Input: part model. Units: mm. Frame: model coordinates. Face numbers are marked on the shaded views. A direction names the side the tool comes from. Give positions to 0.01 mm unless a question says otherwise; leave off trailing zeros. Loops run counter-clockwise (first coordinate to the right, second up) from the corner with the lowest first, then second, coordinate; pieces in that order, holes last. Notation, with made-up numbers: (69.5, -36) -> (94.5, -36) arc R8 cw to (94.5, -26) -> close; hole circle Ø11 at (38.5, 25). An arc over 180 degrees is marked (long way). One line per question, with ' | ' between items.
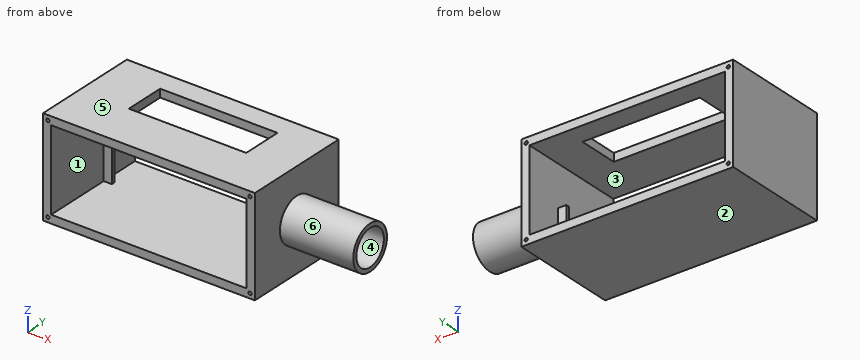
from build123d import *

# Parameters (mm, degrees)
SKETCH1_W           = 130
SKETCH1_H           = 60
BOSS_EXTRUDE1_DEPTH = 67
CUT_EXTRUDE1_REACH  = 69
SKETCH2_W           = 120
SKETCH2_H           = 50
SKETCH4_W           = 27.738428507
SKETCH4_H           = 2
BOSS_EXTRUDE2_DEPTH = 5
SKETCH5_W           = 27.5
SKETCH5_H           = 2
BOSS_EXTRUDE3_DEPTH = 5
CUT_EXTRUDE2_REACH  = 62
SKETCH6_W           = 72
SKETCH6_H           = 25
CUT_EXTRUDE3_REACH  = 69
SKETCH8_R           = 1
SKETCH9_R           = 13.5
BOSS_EXTRUDE4_DEPTH = 45
SKETCH10_R          = 11
CUT_EXTRUDE4_DEPTH  = 45


with BuildPart() as part:
    # Sketch1 → Boss-Extrude1 (new body)
    with BuildSketch(Plane(origin=(0, 0, 0), x_dir=(1, 0, 0), z_dir=(0, 1, 0))):
        Rectangle(SKETCH1_W, SKETCH1_H)
    extrude(amount=BOSS_EXTRUDE1_DEPTH)

    # Sketch2 → Cut-Extrude1 (cut, up to next)
    with BuildSketch(Plane(origin=(0, 67, 0), x_dir=(1, 0, 0), z_dir=(0, 1, 0)), mode=Mode.PRIVATE) as cut_extrude1_sk1:
        Rectangle(SKETCH2_W, SKETCH2_H)
    cut_extrude1_tool1 = extrude(cut_extrude1_sk1.sketch, amount=-CUT_EXTRUDE1_REACH, mode=Mode.PRIVATE) & part.part
    add(cut_extrude1_tool1.solids().sort_by_distance((0, 67, 0))[0], mode=Mode.SUBTRACT)

    # Sketch4 → Boss-Extrude2 (add)
    with BuildSketch(Plane.ZY.offset(-60)):
        with Locations((-13.630785747, 43)):
            Rectangle(SKETCH4_W, SKETCH4_H)
    extrude(amount=BOSS_EXTRUDE2_DEPTH)

    # Sketch5 → Boss-Extrude3 (add)
    with BuildSketch(Plane(origin=(-60, 0, 0), x_dir=(0, 0, -1), z_dir=(1, 0, 0))):
        with Locations((13.75, 43)):
            Rectangle(SKETCH5_W, SKETCH5_H)
    extrude(amount=BOSS_EXTRUDE3_DEPTH)

    # Sketch6 → Cut-Extrude2 (cut, up to next)
    with BuildSketch(Plane.XY.offset(30), mode=Mode.PRIVATE) as cut_extrude2_sk1:
        with Locations((1.435854944, 41.5)):
            Rectangle(SKETCH6_W, SKETCH6_H)
    cut_extrude2_tool1 = extrude(cut_extrude2_sk1.sketch, amount=-CUT_EXTRUDE2_REACH, mode=Mode.PRIVATE) & part.part
    add(cut_extrude2_tool1.solids().sort_by_distance((1.435855, 41.5, 30))[0], mode=Mode.SUBTRACT)

    # Sketch8 → Cut-Extrude3 (cut, up to next)
    with BuildSketch(Plane(origin=(0, 67, 0), x_dir=(1, 0, 0), z_dir=(0, 1, 0)), mode=Mode.PRIVATE) as cut_extrude3_sk1:
        with Locations((-62, 27)):
            Circle(SKETCH8_R)
    cut_extrude3_tool1 = extrude(cut_extrude3_sk1.sketch, amount=-CUT_EXTRUDE3_REACH, mode=Mode.PRIVATE) & part.part
    add(cut_extrude3_tool1.solids().sort_by_distance((-62, 67, -27))[0], mode=Mode.SUBTRACT)
    # Sketch8 → Cut-Extrude3 (cut, up to next)
    with BuildSketch(Plane(origin=(0, 67, 0), x_dir=(1, 0, 0), z_dir=(0, 1, 0)), mode=Mode.PRIVATE) as cut_extrude3_sk2:
        with Locations((62, 27)):
            Circle(SKETCH8_R)
    cut_extrude3_tool2 = extrude(cut_extrude3_sk2.sketch, amount=-CUT_EXTRUDE3_REACH, mode=Mode.PRIVATE) & part.part
    add(cut_extrude3_tool2.solids().sort_by_distance((62, 67, -27))[0], mode=Mode.SUBTRACT)
    # Sketch8 → Cut-Extrude3 (cut, up to next)
    with BuildSketch(Plane(origin=(0, 67, 0), x_dir=(1, 0, 0), z_dir=(0, 1, 0)), mode=Mode.PRIVATE) as cut_extrude3_sk3:
        with Locations((-62, -27)):
            Circle(SKETCH8_R)
    cut_extrude3_tool3 = extrude(cut_extrude3_sk3.sketch, amount=-CUT_EXTRUDE3_REACH, mode=Mode.PRIVATE) & part.part
    add(cut_extrude3_tool3.solids().sort_by_distance((-62, 67, 27))[0], mode=Mode.SUBTRACT)
    # Sketch8 → Cut-Extrude3 (cut, up to next)
    with BuildSketch(Plane(origin=(0, 67, 0), x_dir=(1, 0, 0), z_dir=(0, 1, 0)), mode=Mode.PRIVATE) as cut_extrude3_sk4:
        with Locations((62, -27)):
            Circle(SKETCH8_R)
    cut_extrude3_tool4 = extrude(cut_extrude3_sk4.sketch, amount=-CUT_EXTRUDE3_REACH, mode=Mode.PRIVATE) & part.part
    add(cut_extrude3_tool4.solids().sort_by_distance((62, 67, 27))[0], mode=Mode.SUBTRACT)

    # Sketch9 → Boss-Extrude4 (add)
    with BuildSketch(Plane(origin=(65, 0, 0), x_dir=(0, 0, -1), z_dir=(1, 0, 0))):
        with Locations((0, 33.5)):
            Circle(SKETCH9_R)
    extrude(amount=BOSS_EXTRUDE4_DEPTH)

    # Sketch10 → Cut-Extrude4 (cut)
    with BuildSketch(Plane(origin=(110, 0, 0), x_dir=(0, 0, -1), z_dir=(1, 0, 0))):
        with Locations((0, 33.5)):
            Circle(SKETCH10_R)
    extrude(amount=-CUT_EXTRUDE4_DEPTH, mode=Mode.SUBTRACT)


solid = part.part
1. Section query A-A (z = 18.5). Output: boundary loops of the cut face in (x, y).
Determined:
outline: (-65, 0) -> (-60, 0) -> (-60, 67) -> (-65, 67) -> close; (60, 0) -> (65, 0) -> (65, 67) -> (60, 67) -> close
2. Pin query (flat end, axial travel): P1, Ø4, axis at y = 45.5, z = 27, coming from the +X side; P2, Ø1.5, axis at x = -56.5, z = -16, coming from the -Y side; P3, Ø1.5, axis at x = -56.5, z = -16, coming from the +Y side. Return the tip coordinate at first contact, or that it passes through.
Determined:
P1: stops at x = 65 | P2: stops at y = 42 | P3: stops at y = 44
3. Pull-direction query (Y, two-part tool) for the marked faces 4, 5 and 6; classes: pulls with the +Y half, pulls with the -Y half, needs draft (parallel to the pull), parting line crosses it, or undercut.
Determined:
face 4: undercut | face 5: needs draft | face 6: parting line crosses it
4. Section query B-B (y = 6.5). Output: boundary loops of the cut face in (x, z), then the cut area to 3 significant figures.
Determined:
outline: (-65, -30) -> (65, -30) -> (65, 30) -> (-65, 30) -> close; hole circle Ø2 at (-62, -27); hole circle Ø2 at (-62, 27); hole (-60, -25) -> (60, -25) -> (60, 25) -> (-60, 25) -> close; hole circle Ø2 at (62, -27); hole circle Ø2 at (62, 27) | area: 1,790 mm2
5. Reachability of the marked faces 1, 2 and 3 from +Z, -Z, +X, -X, +Y, -Y: full face, straight path, thin tool, end or side. Return the list, or none.
Determined:
face 1: none | face 2: -Z, +X, -X, +Y, -Y | face 3: +Y, -Y
6. Ray query, line 1 along Z through (x, y) = (-62, 15); line 2 along X through (y, z) = (33, 27); line 3 along X through (y, z) = (19, -19). Return the intervals inside material, ascending. Write a range as from..to.
Determined:
line 1: z = -30..-28, -26..26, 28..30 | line 2: x = -65..-63, -61..-34.56, 37.44..61, 63..65 | line 3: x = -65..-60, 60..65
7. Section query C-C (x = 32.5). Output: boundary loops of the cut face in (y, z), then the cut area to 3 significant figures.
Determined:
outline: (0, -30) -> (67, -30) -> (67, -25) -> (0, -25) -> close; (0, 25) -> (29, 25) -> (29, 30) -> (0, 30) -> close; (54, 25) -> (67, 25) -> (67, 30) -> (54, 30) -> close | area: 545 mm2
8. Section query D-D (y = 25.5). Output: boundary loops of the cut face in (x, z).
Determined:
outline: (-65, -30) -> (65, -30) -> (65, -10.87) -> (110, -10.87) -> (110, -7.55) -> (65, -7.55) -> (65, 7.55) -> (110, 7.55) -> (110, 10.87) -> (65, 10.87) -> (65, 30) -> (-65, 30) -> close; hole circle Ø2 at (-62, -27); hole circle Ø2 at (-62, 27); hole (-60, -25) -> (60, -25) -> (60, 25) -> (-60, 25) -> close; hole circle Ø2 at (62, -27); hole circle Ø2 at (62, 27)
